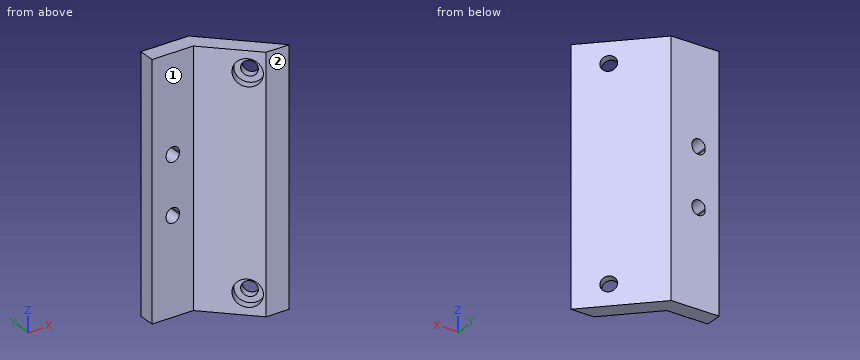
```python
from build123d import *

# Parameters (mm, degrees)
SALIENTE_EXTRUIR1_DEPTH      = 30
SALIENTE_EXTRUIR1_DEPTH_BACK = 30
CROQUIS2_R                   = 1.8
CORTAR_EXTRUIR1_DEPTH        = 4
CROQUIS2_3_R                 = 3.2
CROQUIS2_3_R_2               = 1.8
CORTAR_EXTRUIR2_DEPTH        = 2
CORTAR_EXTRUIR3_DEPTH        = 4


with BuildPart() as part:
    # Croquis1 → Saliente-Extruir1 (new body, two sides)
    with BuildSketch(Plane.XY) as saliente_extruir1_sk:
        Polygon((0, 0), (-14.424978336, 14.424978336), (-26.081832586, 14.424978336), (-26.081832586, 10.424978336), (-16.081832586, 10.424978336), (-5.656854249, 0), align=None)
    extrude(amount=SALIENTE_EXTRUIR1_DEPTH)
    extrude(saliente_extruir1_sk.sketch, amount=-SALIENTE_EXTRUIR1_DEPTH_BACK)

    # Croquis2 → Cortar-Extruir1 (cut)
    with BuildSketch(Plane(origin=(-2.828427125, -2.828427125, 0), x_dir=(-0.707106781, 0.707106781, 0), z_dir=(-0.707106781, -0.707106781, 0))):
        with Locations((7.703145751, -25)):
            Circle(CROQUIS2_R)
        with Locations((7.703145751, 25)):
            Circle(CROQUIS2_R)
    extrude(amount=-CORTAR_EXTRUIR1_DEPTH, mode=Mode.SUBTRACT)

    # Croquis2<3> → Cortar-Extruir2 (cut)
    with BuildSketch(Plane(origin=(-2.828427125, -2.828427125, 0), x_dir=(-0.707106781, 0.707106781, 0), z_dir=(-0.707106781, -0.707106781, 0))):
        with Locations((7.703145751, 25)):
            Circle(CROQUIS2_3_R)
        with Locations((7.703145751, 25)):
            Circle(CROQUIS2_3_R_2, mode=Mode.SUBTRACT)
        with Locations((7.703145751, -25)):
            Circle(CROQUIS2_3_R)
        with Locations((7.703145751, -25)):
            Circle(CROQUIS2_3_R_2, mode=Mode.SUBTRACT)
    extrude(amount=-CORTAR_EXTRUIR2_DEPTH, mode=Mode.SUBTRACT)

    # Croquis3 → Cortar-Extruir3 (cut)
    with BuildSketch(Plane(origin=(0, 14.424978336, 0), x_dir=(1, 0, 0), z_dir=(0, 1, 0))):
        with BuildLine():
            Line((-19.481832586, 7.075), (-19.481832586, 6.75))
            ThreePointArc((-19.481832586, 6.75), (-21.081832586, 5.15), (-22.681832586, 6.75))
            Line((-22.681832586, 6.75), (-22.681832586, 7.075))
            ThreePointArc((-22.681832586, 7.075), (-21.081832586, 8.675), (-19.481832586, 7.075))
        make_face()
        with BuildLine():
            Line((-19.481832586, -7.075), (-19.481832586, -6.75))
            ThreePointArc((-19.481832586, -6.75), (-21.081832586, -5.15), (-22.681832586, -6.75))
            Line((-22.681832586, -6.75), (-22.681832586, -7.075))
            ThreePointArc((-22.681832586, -7.075), (-21.081832586, -8.675), (-19.481832586, -7.075))
        make_face()
    extrude(amount=-CORTAR_EXTRUIR3_DEPTH, mode=Mode.SUBTRACT)


solid = part.part
```
For this review, take the finished solid that the model builds, in its own axes (mm). Face numbers are marked on the shaded views. A direction names the side the tool comes from. Round coordinates to 2 decimals unless told otherwise and drop trailing zeros. Write each loop counter-clockwise with the first axis right and the second up, starting at its lowest first coordinate (ties: lowest second). Pieces come first, ordered by that corner, then holes. Notation, with made-up numbers: (7.25, 26) - (22.25, 26) arc R20 cw to (22.25, 57) - close; hole circle Ø7 at (23.25, 82). An arc over 180 degrees is marked (long way). Answer as CSV lines item,"result". Start each with the question number.
(1) Add section A-A, the plane y = 13.25. State the section outline as (x, z) points (3 decimals), plus the area to 3 significant figures.
(2) For pin 1 (12 mm diameter, centred on x = -17, z = -20.5, fed in from -Y); pin 2 (6 mm diameter, centred on x = -17, z = 12, fed in from -Y); pin 3 (6 mm diameter, centred on y = 10, z = -20.5, fed in from +X); pin 4 (1 mm diameter, centred on x = -19.5, y = 9, fed in from -Z), all flat-tipped, find the tip position at first contact; note any pin that passes through.
(3) Machinability: for the marked faces 1 and 2, which of the approach directions +Z, -Z, +X, -X, +Y, -Y give a long, thin tool a straight path to every point of the face, cutting with its end or side? Answer none if there is none.
(4) Add section D-D, the plane y = 8. State the section outline as (x, z) points.
(5) Add section C-C, the plane x = -18. State the section outline as (y, z) points.
(6) For line 1 (Y direction, x = -18.25, z = 8.5); line 2 (X direction, y = 7.5, z = 2.5); line 3 (X direction, y = 8.25, z = 4), list the stretches that pass through material, from the lowest coordinate up.
(7) Add section B-B, the plane z = 21. State the section outline as (x, y) points, plus the area to 3 significant figures.
From the geometry:
1,outline,"(-26.082, -30) - (-13.25, -30) - (-13.25, 30) - (-26.082, 30) - close; hole (-22.682, -7.075) arc R1.6 ccw to (-19.482, -7.075) - (-19.482, -6.75) arc R1.6 ccw to (-22.682, -6.75) - close; hole (-22.682, 6.75) arc R1.6 ccw to (-19.482, 6.75) - (-19.482, 7.075) arc R1.6 ccw to (-22.682, 7.075) - close"
1,area,"752 mm²"
2,pin 1,"stops at y = 5.34"
2,pin 2,"stops at y = 8.34"
2,pin 3,"stops at x = -7"
2,pin 4,"passes through"
3,face 1,"+Z, -Z, -X, -Y"
3,face 2,"+Z, -Z, +X, -X, -Y"
4,outline,"(-13.66, -30) - (-8, -30) - (-8, 30) - (-13.66, 30) - close"
5,outline,"(10.42, -30) - (14.42, -30) - (14.42, 30) - (10.42, 30) - close"
6,line 1,"y = 10.42 to 14.42"
6,line 2,"x = -13.16 to -7.5"
6,line 3,"x = -13.91 to -8.25"
7,outline,"(-26.08, 10.42) - (-16.08, 10.42) - (-5.66, 0) - (0, 0) - (-14.42, 14.42) - (-26.08, 14.42) - close"
7,area,"114 mm²"
